```python
from build123d import *

# Parameters (mm, degrees)
F1_DEPTH = 63.5
F2_DEPTH = 25.4
F3_DEPTH = 7.9375
F5_R     = 6.35


with BuildPart() as f1:
    # F0 (on Front) → F1 (new body, symmetric)
    with BuildSketch(Plane.XZ):
        Polygon((-41.275, 9.525), (-41.275, -9.525), (41.275, -9.525), (41.275, 9.525), (22.225, 9.525), align=None)
    extrude(amount=F1_DEPTH, both=True)

    # F0 (on Front) → F2 (join, symmetric)
    with BuildSketch(Plane.XZ):
        Polygon((85.725, 61.9252), (60.325, 61.9252), (60.325, 42.8752), (85.725, 42.8752), (85.725, 52.3875), align=None)
        with BuildLine():
            Line((22.225, 9.525), (41.275, 9.525))
            Line((41.275, 9.525), (41.275, 27.0002))
            ThreePointArc((41.275, 27.0002), (45.92468, 38.22552), (57.15, 42.8752))
            Line((57.15, 42.8752), (60.325, 42.8752))
            Line((60.325, 42.8752), (60.325, 61.9252))
            Line((60.325, 61.9252), (57.15, 61.9252))
            add(Edge.make_bspline(
                [(55.092977, 61.86457), (55.785837, 61.89427), (56.471675, 61.914556), (57.15, 61.9252)],
                knots=[109.502305, 109.502305, 109.502305, 109.502305, 111.504536, 111.504536, 111.504536, 111.504536], degree=3))
            ThreePointArc((55.092977, 61.86457), (31.737433, 50.957601), (22.225, 27.0002))
            Line((22.225, 27.0002), (22.225, 9.525))
        make_face()
    extrude(amount=F2_DEPTH, both=True)

    # F0 (on Front) → F3 (join, symmetric)
    with BuildSketch(Plane.XZ):
        with BuildLine():
            add(Edge.make_bspline(
                [(-41.275, 9.525), (-41.696727, 30.455088), (17.200338, 60.240237), (55.092977, 61.86457)],
                knots=[0, 0, 0, 0, 109.502305, 109.502305, 109.502305, 109.502305], degree=3))
            Line((-41.275, 9.525), (22.225, 9.525))
            Line((22.225, 9.525), (22.225, 27.0002))
            ThreePointArc((22.225, 27.0002), (31.737433, 50.957601), (55.092977, 61.86457))
        make_face()
    extrude(amount=F3_DEPTH, both=True)

    # F0 (on Front) → F4 (revolve)
    with BuildSketch(Plane.XZ):
        Polygon((85.725, 66.675), (85.725, 61.9252), (85.725, 52.3875), (85.725, 42.8752), (85.725, 38.1), (111.125, 38.1), (111.125, 66.675), align=None)
    revolve(axis=Axis((85.725, 0, 47.63135), (0, 0, -1)))

    # F5
    f5_edges = [f1.edges().sort_by_distance(p)[0] for p in [
        (-41.275, -63.5, 0),
        (41.275, 63.5, 0),
        (41.275, -63.5, 0),
        (-41.275, 63.5, 0),
    ]]
    fillet(f5_edges, radius=F5_R)


solid = f1.part
```
The listing builds one solid part. Answer for the finished solid, in the listing's coordinates (mm). A direction names the side the tool comes from. Give positions to 0.01 mm unless a question says otherwise; leave off trailing zeros. Loops run counter-clockwise (first coordinate to the right, second up) from the corner with the lowest first, then second, coordinate; pieces in that order, holes last. Notation, with made-up numbers: (89, 2) - (116, 2) arc R7 cw to (116, 10) - close; hole circle Ø5 at (39.5, 30). An arc over 180 degrees is marked (long way). Return JSON: item names as keys, results as strings. Group by question number.
1. Determine the mould class of faces 1 (the flat face through (60, 2, 42.875)), 2 (the flat face through (-1, -1, -9.525)), 3 (the cylindrical face through (39.464, -61.59, 0.133)) for opening direction X: pulls with the +X half, pulls with the -X half, needs draft (parallel to the pull), parting line crosses it, or undercut.
2. Straight lines are drawn through the part: line 1 (Y direction, x = 86, z = 47); line 2 (Z direction, x = 5.5, y = 18.5) (3 decimals); line 3 (Z direction, x = 94, y = 0) (3 decimals). For each, find the intervals that lie inside material, in ascending order. Write a range as [from, to].
3. Given pin 1 Ø19 at (y, z) = (20.5, 20) entering from -X (3 decimals); pin 2 Ø19 at (y, z) = (-15, 21) entering from -X; pin 3 Ø12 at (y, z) = (8.5, 37) entering from +X, each flat-ended and moving along its own axis, determine where each tip first touches the part or whether it passes through.
4. Find section B-B (x = 65). Write down the section's boundary in (y, z) (1 decimal), then the cut area to 3 significant figures.
5. Find section A-A (z = -2.5). Write down the section's boundary in (x, y) (3 decimals).
6. Find section C-C (y = -53.5). Write down the section's boundary in (x, z) (3 decimals), then the cut area to 3 significant figures.
7. Which of the six approach directions +Z, -Z, +X, -X, +Y, -Y give full straight-line access (tool end or side, diameter ignored) to faces 4 (the flat face through (-3, -7.938, 30)), 5 (the cylindrical face through (31.992, 16.547, 51.225)), 6 (the flat face through (46, -25.4, 42))?
Verdict:
{
 "1": {"face 1": "undercut", "face 2": "needs draft", "face 3": "pulls with the +X half"},
 "2": {"line 1": "y = [-25.4, 25.4]", "line 2": "z = [-9.525, 9.525]", "line 3": "z = [38.1, 66.675]"},
 "3": {"pin 1": "stops at x = 22.225", "pin 2": "stops at x = -40.3", "pin 3": "stops at x = 110.99"},
 "4": {"outline": "(-25.4, 42.9) - (-14.7, 42.9) - (-14.7, 38.1) - (14.7, 38.1) - (14.7, 42.9) - (25.4, 42.9) - (25.4, 61.9) - (14.7, 61.9) - (14.7, 66.7) - (-14.7, 66.7) - (-14.7, 61.9) - (-25.4, 61.9) - close", "area": "1,250 mm^2"},
 "5": {"outline": "(-41.275, -57.15) arc R6.35 ccw to (-34.925, -63.5) - (34.925, -63.5) arc R6.35 ccw to (41.275, -57.15) - (41.275, 57.15) arc R6.35 ccw to (34.925, 63.5) - (-34.925, 63.5) arc R6.35 ccw to (-41.275, 57.15) - close"},
 "6": {"outline": "(-41.275, -9.525) - (41.275, -9.525) - (41.275, 9.525) - (-41.275, 9.525) - close", "area": "1,570 mm^2"},
 "7": {"face 4": "+Z, -X, -Y", "face 5": "+Z, -X, +Y", "face 6": "+Z, +X, -X, -Y"}
}
